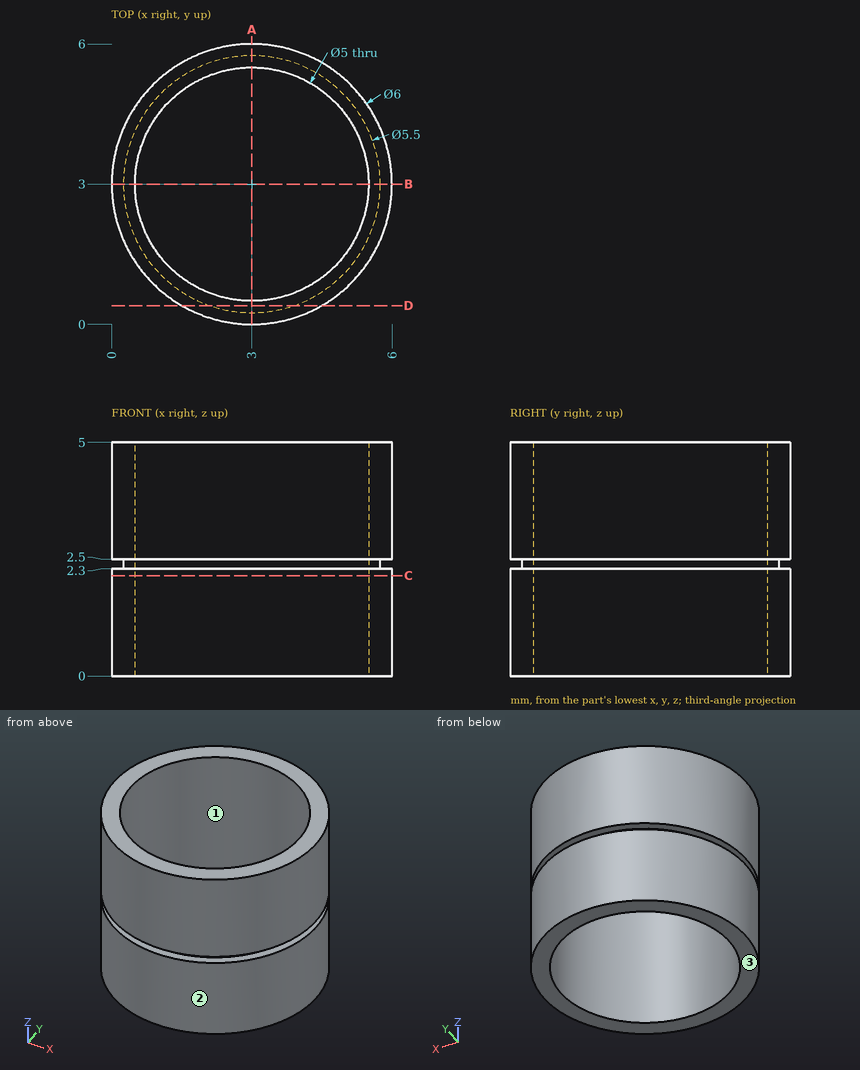
Geometry check sheet. Reference: drawing and pictorial views, mm from the part's lowest x, y, z. Round coordinates to 2 decimals unless told otherwise and drop trailing zeros. Loops run counter-clockwise (first coordinate to the right, second up) from the corner with the lowest first, then second, coordinate; pieces in that order, holes last. Notation, with made-up numbers: (88.5, -8.75) -> (133.5, -8.75) arc R30 cw to (133.5, 28.25) -> close; hole circle Ø3 at (80.25, 28). An arc over 180 degrees is marked (long way). Use a Markdown table: item, result.
(1) Mould release check, pull along X, two halves, no side actions. Record for the marked faces 1, 2 and 3: released by +X, released by -X, zero draft, split by the parting line, or undercut.
Calculated:
| item | result |
|---|---|
| face 1 | undercut |
| face 2 | split by the parting line |
| face 3 | zero draft |
(2) Scan lines: probe 1 along Y at (x, z) = (2.95, 1.1); probe 2 along Y at (x, z) = (3, 2.45); probe 3 along X at (y, z) = (3.7, 1.2). Record each from-to range of solid material in increasing order.
Calculated:
| item | result |
|---|---|
| probe 1 | 0 to 0.5, 5.5 to 6 |
| probe 2 | 0.25 to 0.5, 5.5 to 5.75 |
| probe 3 | 0.08 to 0.6, 5.4 to 5.92 |
(3) Go/stop test with a flat-tipped pin: P1, Ø1.5, axis at x = 4, z = 1, coming from the +Y side. Record where the tip stops, or that it passes through.
Calculated:
| item | result |
|---|---|
| P1 | y = 5.99 |
(4) Sectioned sample at D-D (y = 0.4). Enter the section's corners in (x, z), then the cut area to 3 significant figures.
Calculated:
| item | result |
|---|---|
| outline | (1.5, 0) -> (4.5, 0) -> (4.5, 2.3) -> (3.9, 2.3) -> (3.9, 2.5) -> (4.5, 2.5) -> (4.5, 5) -> (1.5, 5) -> (1.5, 2.5) -> (2.1, 2.5) -> (2.1, 2.3) -> (1.5, 2.3) -> close |
| area | 14.7 mm² |
(5) Sectioned sample at C-C (z = 2.15). Enter the section's corners in (x, y).
Calculated:
| item | result |
|---|---|
| outline | circle Ø6 at (3, 3); hole circle Ø5 at (3, 3) |
(6) Sectioned sample at A-A (x = 3). Enter the section's corners in (y, z), then the cut area to 3 significant figures.
Calculated:
| item | result |
|---|---|
| outline | (0, 0) -> (0.5, 0) -> (0.5, 5) -> (0, 5) -> (0, 2.5) -> (0.25, 2.5) -> (0.25, 2.3) -> (0, 2.3) -> close; (5.5, 0) -> (6, 0) -> (6, 2.3) -> (5.75, 2.3) -> (5.75, 2.5) -> (6, 2.5) -> (6, 5) -> (5.5, 5) -> close |
| area | 4.90 mm² |
